Geometry: final body of the model. Coordinates: model frame, mm. Face numbers are marked on the shaded views. A direction names the side the tool comes from. Coordinates: 2 decimals unless noted, no trailing zeros. Write each loop counter-clockwise with the first axis right and the second up, starting at its lowest first coordinate (ties: lowest second). Pieces come first, ordered by that corner, then holes. Notation, with made-up numbers: (-38.75, 13) -> (-30.75, 13) arc R19 cw to (-30.75, 43) -> close; hole circle Ø7 at (43, 48.25). An arc over 180 degrees is marked (long way). One line per item, written item: value.
```python
from build123d import *

# Parameters (mm, degrees)
CUT_EXTRUDE1_DEPTH      = 11.464224768
CUT_EXTRUDE1_DEPTH_BACK = 5
CHAMFER1_SIZE           = 0.1


with BuildPart() as part:
    # Sketch1 → Revolve1 (revolve)
    with BuildSketch(Plane.XY, mode=Mode.PRIVATE) as revolve1_sk:
        Polygon((3, 0), (5.5, 0), (5.5, 2), (4.5, 2), (4.5, 7), (3, 7), align=None)
    revolve(revolve1_sk.sketch.rotate(Axis((0, 0, 0), (0, 1, 0)), 90), axis=Axis((0, 0, 0), (0, 1, 0)))

    # Sketch2 → Cut-Extrude1 (cut, two sides: drawn at the far end of the back side and taken through both)
    with BuildSketch(Plane(origin=(0, 7, 0), x_dir=(1, 0, 0), z_dir=(0, 1, 0)).offset(-CUT_EXTRUDE1_DEPTH_BACK)):
        with BuildLine():
            Line((-4, 2.061552813), (-4, -2.061552813))
            ThreePointArc((-4, -2.061552813), (-4.5, 0), (-4, 2.061552813))
        make_face()
        with BuildLine():
            Line((4, 2.061552813), (4, -2.061552813))
            ThreePointArc((4, -2.061552813), (4.5, 0), (4, 2.061552813))
        make_face()
    extrude(amount=CUT_EXTRUDE1_DEPTH + CUT_EXTRUDE1_DEPTH_BACK, mode=Mode.SUBTRACT)

    # Chamfer1
    chamfer1_edges = [part.edges().sort_by_distance(p)[0] for p in [
        (0, 7, 4.5),
        (0, 7, -4.5),
        (4, 7, 0),
        (-4, 7, 0),
        (0, 0, 5.5),
    ]]
    chamfer(chamfer1_edges, length=CHAMFER1_SIZE)


solid = part.part
```
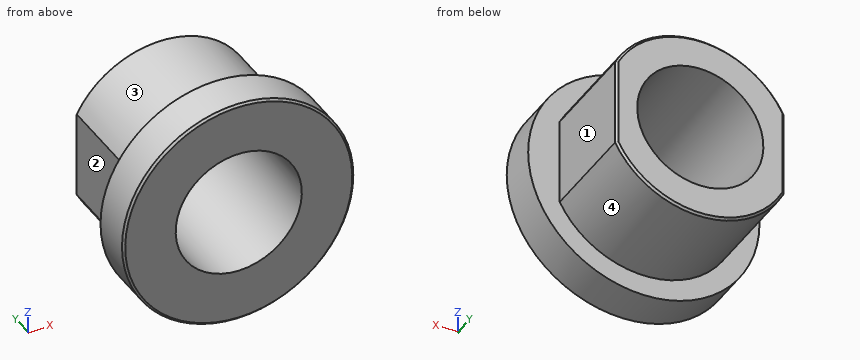
(1) First-contact query: pin 1 (3.5 mm diameter, centred on y = 4, z = -0.5, fed in from -X); pin 2 (2 mm diameter, centred on y = 4, z = 4.5, fed in from +X); pin 3 (1 mm diameter, centred on x = -1, y = 6.5, fed in from +Z). Flat tips, straight axial feed; report the tip coordinate or a pass-through.
Responses:
pin 1: stops at x = -4
pin 2: stops at x = 2.83
pin 3: stops at z = 4.47
(2) Section D-D (y = 0.75). Return the cut outline in (x, z).
Responses:
outline: circle Ø11 at (0, 0); hole circle Ø6 at (0, 0)
(3) Section A-A (x = 0). Return the cut outline in (y, z), then the cut area to 3 significant figures.
Responses:
outline: (0, -5.4) -> (0.1, -5.5) -> (2, -5.5) -> (2, -4.5) -> (6.9, -4.5) -> (7, -4.4) -> (7, -3) -> (0, -3) -> close; (0, 3) -> (7, 3) -> (7, 4.4) -> (6.9, 4.5) -> (2, 4.5) -> (2, 5.5) -> (0.1, 5.5) -> (0, 5.4) -> close
area: 25.0 mm2
(4) Reachability of the marked faces 1, 2, 3 and 4 from +Z, -Z, +X, -X, +Y, -Y: full face, straight path, thin tool, end or side. Return the list, or none.
Responses:
face 1: +Z, -Z, +X, +Y
face 2: +Z, -Z, -X, +Y
face 3: +Z, +Y
face 4: -Z, +Y
(5) Line query: line 1 (X direction, y = 5, z = 0); line 2 (Y direction, x = 4, z = 3); line 3 (X direction, y = 6.25, z = -1). Output: solid intervals per line, ascending. Write a range as [from, to].
Responses:
line 1: x = [-4, -3], [3, 4]
line 2: y = [0, 2]
line 3: x = [-4, -2.83], [2.83, 4]
(6) Section C-C (y = 6.5). Return the cut outline in (x, z), then the cut area to 3 significant figures.
Responses:
outline: (-4, -2.06) arc R4.5 ccw to (4, -2.06) -> (4, 2.06) arc R4.5 ccw to (-4, 2.06) -> close; hole circle Ø6 at (0, 0)
area: 32.6 mm2
(7) Section B-B (z = 0). Return the cut outline in (x, y), then the cut area to 3 significant figures.
Responses:
outline: (-5.5, 0.1) -> (-5.4, 0) -> (-3, 0) -> (-3, 7) -> (-3.9, 7) -> (-4, 6.9) -> (-4, 2) -> (-5.5, 2) -> close; (3, 0) -> (5.4, 0) -> (5.5, 0.1) -> (5.5, 2) -> (4, 2) -> (4, 6.9) -> (3.9, 7) -> (3, 7) -> close
area: 20.0 mm2
